from build123d import *

# Parameters (mm, degrees)
SKETCH1_R           = 13.716
BOSS_EXTRUDE1_DEPTH = 127
SKETCH2_R           = 10.668
CUT_EXTRUDE1_DEPTH  = 127
SCALE1_SCALE        = 0.735294118
SCALE2_SCALE        = 0.892857143
SCALE3_SCALE        = 1.056338028


with BuildPart() as part:
    # Sketch1 → Boss-Extrude1 (new body)
    with BuildSketch(Plane.XY):
        with Locations((-7.319167791, 4.997022186)):
            Circle(SKETCH1_R)
    extrude(amount=BOSS_EXTRUDE1_DEPTH)

    # Sketch2 → Cut-Extrude1 (cut)
    with BuildSketch(Plane(origin=(0, 0, 0), x_dir=(-1, 0, 0), z_dir=(0, 0, -1))):
        with Locations((7.319167791, 4.997022186)):
            Circle(SKETCH2_R)
    extrude(amount=-CUT_EXTRUDE1_DEPTH, mode=Mode.SUBTRACT)


with BuildPart() as part_1:
    # Scale1: scaled about (-7.319167791, 4.997022186, 63.5)
    add(part.part.scale(SCALE1_SCALE).moved(Location((-1.937426768, 1.322741167, 16.808823529))))


with BuildPart() as part_2:
    # Scale2: scaled about (-7.319167791, 4.997022186, 63.5)
    add(part_1.part.scale(SCALE2_SCALE).moved(Location((-0.784196549, 0.535395234, 6.803571429))))


with BuildPart() as part_3:
    # Scale3: scaled about (-7.319167791, 4.997022186, 63.5)
    add(part_2.part.scale(SCALE3_SCALE).moved(Location((0.412347481, -0.281522377, -3.577464789))))


solid = part_3.part
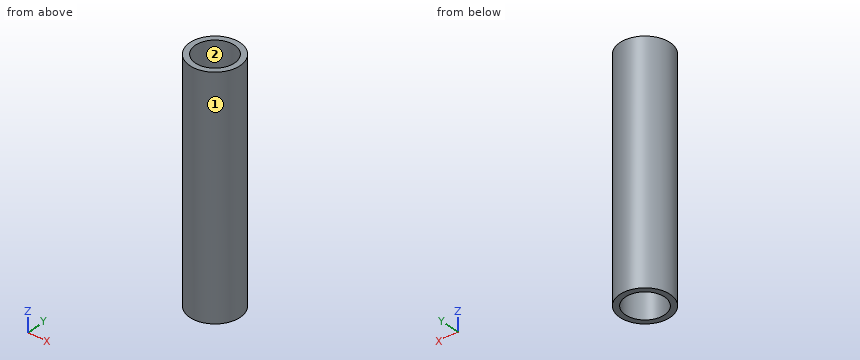
Input: part model. Units: mm. Frame: model coordinates. Face numbers are marked on the shaded views. Coordinates: 2 decimals unless noted, no trailing zeros. Order: outer loops, then holes, each group sorted by start corner. A loop starts at its lowest first (then second) coordinate and runs counter-clockwise, first axis right, second up. Notation, with made-up numbers: M 6.5,28 L 24.5,28 A31 cw 24.5,55 Z; hole C 27.25,11 d5. An arc over 180 degrees is marked long. Write item = value, one per line. Start each with the question number.
(1) Line query: line 1 along Y through (x, z) = (-13.25, 25.5); line 2 along X through (y, z) = (-1.75, 73); line 3 along X through (y, z) = (8.75, 29). Output: solid intervals per line, ascending. Write a range as [from, to].
(2) Section B-B on x = -12.5. Output: boundary loops of the cut face in (y, z).
(3) Pull-direction query (Y, two-part tool) for the marked faces 1 and 2; classes: released by +Y, released by -Y, zero draft, split by the parting line, or undercut.
(4) First-contact query: P1, Ø10, axis at x = -13.5, z = 48, coming from the +Y side; P2, Ø3, axis at x = -1, z = 51.5, coming from the -Y side; P3, Ø5, axis at x = -1.5, z = 60, coming from the -Y side; P4, Ø3, axis at x = -8, y = 0.5, coming from the -Z side. Flat tips, straight axial feed; report the tip coordinate or a pass-through.
(5) Section A-A on y = 0. Output: boundary loops of the cut face in (x, z).
(6) Section C-C on z = 95. Output: boundary loops of the cut face in (x, y), and give its area (3 significant figures).
Result set:
q1.line_1 = [-2.44, 0.57], [9.42, 12.43]
q1.line_2 = [-14.02, -10.35], [-4.28, -0.61]
q1.line_3 = [-16.06, -13.69], [-0.94, 1.42]
q2.outline = M -2.98,19.46 L -0.28,19.46 L -0.28,107.54 L -2.98,107.54 Z; M 10.28,19.46 L 12.97,19.46 L 12.97,107.54 L 10.28,107.54 Z
q3.face_1 = split by the parting line
q3.face_2 = undercut
q4.P1 = 14.44
q4.P2 = -3.2
q4.P3 = -3.92
q4.P4 = through
q5.outline = M -15.41,19.46 L -12.77,19.46 L -12.77,107.54 L -15.41,107.54 Z; M -1.86,19.46 L 0.77,19.46 L 0.77,107.54 L -1.86,107.54 Z
q6.outline = C -7.32,5 d19.02; hole C -7.32,5 d14.8
q6.area = 112 mm²
